Can you work these out from the model? Positions are in its coordinate system, mm. A direction names the side the tool comes from. Give positions to 0.01 mm unless a question says otherwise; leave off trailing zeros. Order: outer loops, then holes, each group sorted by start corner. A loop starts at its lowest first (then second) coordinate and runs counter-clockwise, first axis right, second up. Notation, with made-up numbers: M 66,43.5 L 92,43.5 A34 ccw 92,74.5 Z; hole C -27,-4.5 d2. An arc over 180 degrees is marked long. Write each question's results on one line, items separated by ' | '.
from build123d import *

# Parameters (mm, degrees)
SKETCH1_R                           = 4.35
REBAIXO_DE_ENCAIXE_DEPTH            = 2.6
SKETCH14_R                          = 2.45
FURO_DE_ENCAIXE_SERVO_DEPTH         = 3
SKETCH5_R                           = 10.55
SKETCH5_R_2                         = 1.35
BASE_REDONDA_DEPTH                  = 2
SKETCH8_R                           = 3.425
SKETCH8_R_2                         = 2.925
RESSALTO_DEPTH                      = 0.8
SKETCH9_R                           = 0.75
FUROS_DE_FIXA_O_CARGA_REDONDO_DEPTH = 16.612975373


with BuildPart() as part:
    # Sketch1 → Rebaixo de Encaixe (new body)
    with BuildSketch(Plane(origin=(0, 0, 0), x_dir=(1, 0, 0), z_dir=(0, 1, 0))):
        with Locations(Location((0, 0, 0), (0, 0, 270))):
            Circle(SKETCH1_R)
    extrude(amount=REBAIXO_DE_ENCAIXE_DEPTH)

    # Sketch14 → Furo de Encaixe - Servo (cut)
    with BuildSketch(Plane.XZ):
        with Locations(Location((0, 0, 0), (0, 0, 270))):
            Circle(SKETCH14_R)
    extrude(amount=-FURO_DE_ENCAIXE_SERVO_DEPTH, mode=Mode.SUBTRACT)

    # Sketch5 → Base Redonda (add)
    with BuildSketch(Plane(origin=(0, 2.6, 0), x_dir=(1, 0, 0), z_dir=(0, 1, 0))):
        with Locations(Location((0, 0, 0), (0, 0, 270))):
            Circle(SKETCH5_R)
        with Locations(Location((0, 0, 0), (0, 0, 270))):
            Circle(SKETCH5_R_2, mode=Mode.SUBTRACT)
    extrude(amount=BASE_REDONDA_DEPTH)

    # Sketch8 → Ressalto (add)
    with BuildSketch(Plane(origin=(0, 4.6, 0), x_dir=(1, 0, 0), z_dir=(0, 1, 0))):
        with Locations(Location((0, 0, 0), (0, 0, 270))):
            Circle(SKETCH8_R)
        with Locations(Location((0, 0, 0), (0, 0, 270))):
            Circle(SKETCH8_R_2, mode=Mode.SUBTRACT)
    extrude(amount=RESSALTO_DEPTH)

    # Sketch9 → Furos de Fixação - Carga Redondo (cut, through all)
    with BuildSketch(Plane(origin=(0, 4.6, 0), x_dir=(1, 0, 0), z_dir=(0, 1, 0))):
        with Locations(Location((0, 7.15, 0), (0, 0, 270))):
            Circle(SKETCH9_R)
        with Locations(Location((3.5, 7.15, 0), (0, 0, 270))):
            Circle(SKETCH9_R)
        with Locations(Location((-3.5, 7.15, 0), (0, 0, 270))):
            Circle(SKETCH9_R)
        with Locations(Location((7.15, 3.5, 0), (0, 0, 270))):
            Circle(SKETCH9_R)
        with Locations(Location((7.15, 0, 0), (0, 0, 270))):
            Circle(SKETCH9_R)
        with Locations(Location((7.15, -3.5, 0), (0, 0, 270))):
            Circle(SKETCH9_R)
        with Locations(Location((3.5, -7.15, 0), (0, 0, 270))):
            Circle(SKETCH9_R)
        with Locations(Location((0, -7.15, 0), (0, 0, 270))):
            Circle(SKETCH9_R)
        with Locations(Location((-3.5, -7.15, 0), (0, 0, 270))):
            Circle(SKETCH9_R)
        with Locations(Location((-7.15, -3.5, 0), (0, 0, 270))):
            Circle(SKETCH9_R)
        with Locations(Location((-7.15, 0, 0), (0, 0, 270))):
            Circle(SKETCH9_R)
        with Locations(Location((-7.15, 3.5, 0), (0, 0, 270))):
            Circle(SKETCH9_R)
    extrude(amount=-FUROS_DE_FIXA_O_CARGA_REDONDO_DEPTH, mode=Mode.SUBTRACT)


solid = part.part
(1) Imagine slicing it at C-C, the plane x = -4. Write out the boundary of the cut face in (y, z), plus the area to 3 significant figures.
Data:
outline: M 0,-1.71 L 2.6,-1.71 L 2.6,-6.59 L 4.6,-6.59 L 4.6,6.59 L 2.6,6.59 L 2.6,1.71 L 0,1.71 Z; M 2.6,-9.76 L 4.6,-9.76 L 4.6,-7.71 L 2.6,-7.71 Z; M 2.6,7.71 L 4.6,7.71 L 4.6,9.76 L 2.6,9.76 Z | area: 43.5 mm2
(2) For faces 1 (the face through (-1.1, 2.6, 1.1)), 2 (the face through (-4.165, 3.614, -6.804)), 3 (the face through (-5, 4.6, 0)), which set-ups out of +Z, -Z, +X, -X, +Y, -Y let a thin tool reach every point of the face, with its end or its side?
Data:
face 1: -Y | face 2: +Y, -Y | face 3: +Y
(3) I need wall thicknesses on L1, parallel to X at y = 3.75, z = 0; L2, parallel to Z at x = 6.75, y = 4.3; L3, parallel to Y at x = -4, z = -8.25. Which ranges of each line are inside material? Lowest first, please. Write a range as from..to.
Data:
L1: x = -10.55..-7.9, -6.4..-1.35, 1.35..6.4, 7.9..10.55 | L2: z = -8.11..-4.13, -2.87..-0.63, 0.63..2.87, 4.13..8.11 | L3: y = 2.6..4.6
(4) We'd pull the mould along Z, two halves only. Please class faces 4 (the face through (7.13, 3.586, -7.776)), 5 (the face through (1, 5.4, 3)), 6 (the face through (6.418, 3.614, 3.337)): +Z half, -Z half, draft (parallel to the pull), parting line (faces both ways), or undercut.
Data:
face 4: parting line | face 5: draft | face 6: undercut
(5) Imagine slicing it at D-D, the plane y = 1.05. Write out the boundary of the cut face in (x, z), plus the area to 3 significant figures.
Data:
outline: C 0,0 d8.7; hole C 0,0 d4.9 | area: 40.6 mm2
(6) Will these pins go through, and if not, where does the flat tip stop? P1, Ø2.5, axis at x = -3.5, z = 7.15, coming from the -Y side; P2, Ø2.5, axis at x = 0, z = 7.15, coming from the +Y side.
Data:
P1: stops at y = 2.6 | P2: stops at y = 4.6
(7) Imagine slicing it at A-A, the plane x = 0. Count the separate pieces of the cut face and the enclosed holes in it, plus the area to 3 significant figures.
Data:
separate pieces: 4 | enclosed holes: 0 | area: 41.5 mm2
